Part print with two shaded views. Sizes in mm from the minimum x, y, z corner. A direction names the side the tool comes from. Give positions to 0.01 mm unless a question says otherwise; leave off trailing zeros. Write each loop counter-clockwise with the first axis right and the second up, starting at its lowest first coordinate (ties: lowest second). Pieces come first, ordered by that corner, then holes. Notation, with made-up numbers: (58, 85.5) - (111, 85.5) arc R15 cw to (111, 101.5) - close; hole circle Ø10 at (-20, 87.25). An arc over 180 degrees is marked (long way). Answer as a JSON object with one key per item and string values.
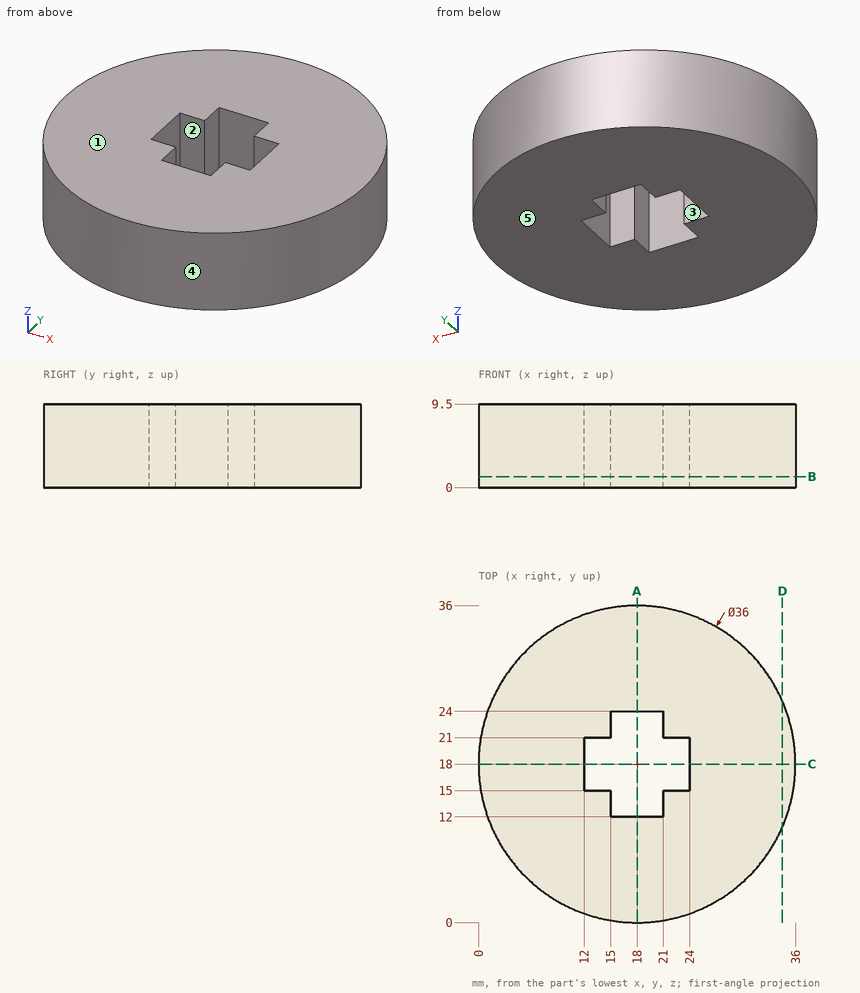
(1) Saw through at B-B, the plane z = 1.25. Give the cut face in (x, y).
Answer key:
{"outline": "circle Ø36 at (18, 18); hole (12, 15) - (15, 15) - (15, 12) - (21, 12) - (21, 15) - (24, 15) - (24, 21) - (21, 21) - (21, 24) - (15, 24) - (15, 21) - (12, 21) - close"}
(2) Saw through at A-A, the plane x = 18. Give the cut face in (y, z), and give its area (3 significant figures).
Answer key:
{"outline": "(0, 0) - (12, 0) - (12, 9.5) - (0, 9.5) - close; (24, 0) - (36, 0) - (36, 9.5) - (24, 9.5) - close", "area": "228 mm²"}
(3) 3-axis set-ups, long thin cutter, end or side, ignore diameter. For the marked faces 1 and 2: which of +Z, -Z, +X, -X, +Y, -Y reach the whole face in a straight line?
Answer key:
{"face 1": "+Z, +X, -X, +Y, -Y", "face 2": "+Z, -Z"}
(4) Probe L1, parallel to X at y = 18.5, z = 6.75; L2, parallel to X at y = 22, z = 0.75. List the from-to ranges inside material, lowest first. Write a range as [from, to].
Answer key:
{"L1": "x = [0.01, 12], [24, 35.99]", "L2": "x = [0.45, 15], [21, 35.55]"}
(5) Pull direction X, two halves, no side cores. Call the marked faces 3, 4 and 5: pulls with the +X half, pulls with the -X half, needs draft (parallel to the pull), parting line crosses it, or undercut.
Answer key:
{"face 3": "undercut", "face 4": "parting line crosses it", "face 5": "needs draft"}
(6) Flat gauge pins, fed straight in: P1, Ø4, axis at y = 27, z = 7.5, coming from the -X side; P2, Ø2, axis at y = 32, z = 8, coming from the -X side; P3, Ø1.5, axis at x = 23, z = 5.5, coming from the -Y side. Where does each tip first touch, or does it go through?
Answer key:
{"P1": "stops at x = 1.42", "P2": "stops at x = 5.55", "P3": "stops at y = 0.51"}
(7) Saw through at D-D, the plane x = 34.5. Give the cut face in (y, z).
Answer key:
{"outline": "(10.81, 0) - (25.19, 0) - (25.19, 9.5) - (10.81, 9.5) - close"}
